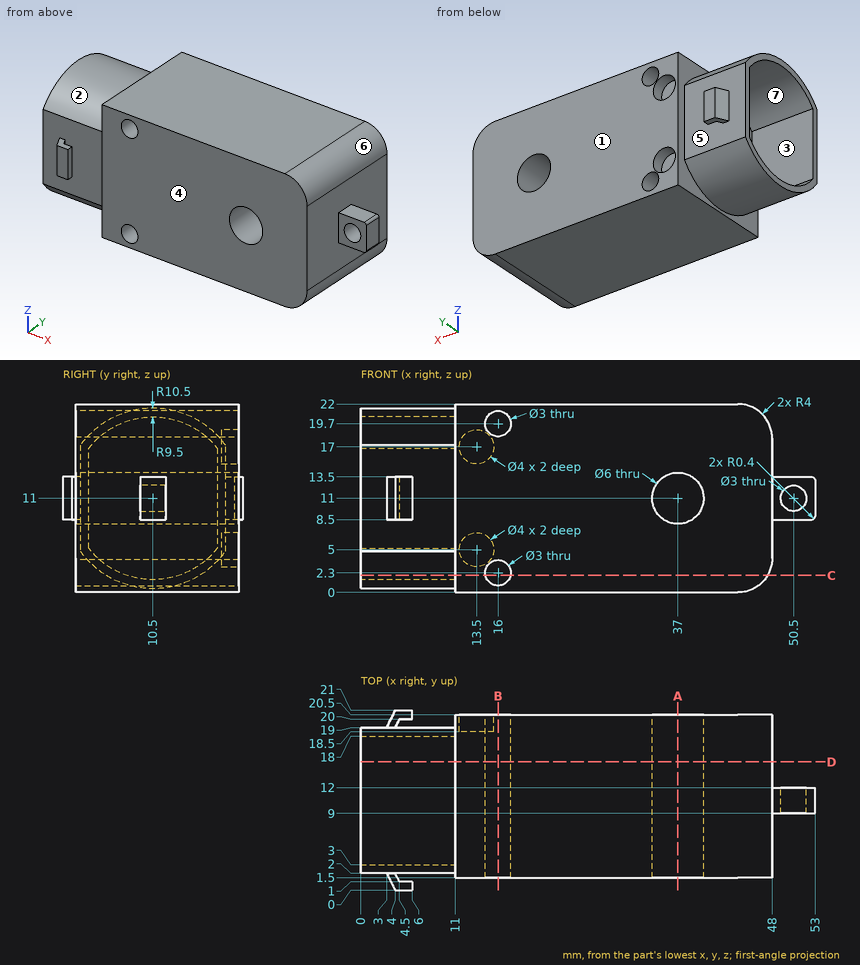
Print and shaded views of the part. All mm, measured from the part's lowest x, y and z. A direction names the side the tool comes from. Coordinates: 2 decimals unless noted, no trailing zeros. Loops run counter-clockwise (first coordinate to the right, second up) from the corner with the lowest first, then second, coordinate; pieces in that order, holes last. Notation, with made-up numbers: (80.5, 38) -> (138.5, 38) arc R27 ccw to (138.5, 76) -> close; hole circle Ø11 at (75, -35.5). An arc over 180 degrees is marked (long way). Use a Markdown table: item, result. Add a question column.
Item 1: Band-saw the part on B-B on x = 16. Write the cut outline in (y, z).
Item 2: Which spindle directions (+Z, -Z, +X, -X, +Y, -Y) get a long thin tool onto all of the face, cutting with end or side? Do the marked faces 1, 2, 3 and 4. Say none if no direction does.
Item 3: Band-saw the part on A-A on x = 37. Write the cut outline in (y, z).
Item 4: Probe probe 1 along X at (y, z) = (11.2, 11); probe 2 along X at (y, z) = (19.2, 17); probe 3 along X at (y, z) = (13.25, 5.25). List the from-to ranges inside material, lowest first.
Item 5: Band-saw the part on D-D on y = 15. Write the cut outline in (x, z).
Item 6: Flat gauge pins, fed straight in: P1, Ø2, axis at x = 13.5, z = 4.5, coming from the +Y side; P2, Ø2.5, axis at x = 51.5, z = 11.5, coming from the +Y side; P3, Ø0.9, axis at x = 51, y = 11, coming from the +Z side. Where does each tip first touch, or does it go through?
Item 7: Band-saw the part on C-C on z = 2. Write the cut outline in (x, y).
Item 8: Pull direction X, two halves, no side cores. Call the marked faces 5, 6 and 7: +X half, -X half, draft (parallel to the pull), parting line (faces both ways), or undercut.
Geometry says:
| question | item | result |
|---|---|---|
| 1 | outline | (1.5, 0) -> (20.5, 0) -> (20.5, 0.8) -> (1.5, 0.8) -> close; (1.5, 3.8) -> (20.5, 3.8) -> (20.5, 18.2) -> (1.5, 18.2) -> close; (1.5, 21.2) -> (20.5, 21.2) -> (20.5, 22) -> (1.5, 22) -> close |
| 2 | face 1 | +Z, -Z, +X, +Y |
| 2 | face 2 | +Z, -X |
| 2 | face 3 | -X |
| 2 | face 4 | +Z, -Z, +X, -Y |
| 3 | outline | (1.5, 0) -> (20.5, 0) -> (20.5, 8) -> (1.5, 8) -> close; (1.5, 14) -> (20.5, 14) -> (20.5, 22) -> (1.5, 22) -> close |
| 4 | probe 1 | 11 to 34, 40 to 49, 52 to 53 |
| 4 | probe 2 | 11 to 11.5, 15.5 to 48 |
| 4 | probe 3 | 11 to 48 |
| 5 | outline | (0, 1.51) -> (11, 1.51) -> (11, 0) -> (44, 0) arc R4 ccw to (48, 4) -> (48, 18) arc R4 ccw to (44, 22) -> (11, 22) -> (11, 20.49) -> (0, 20.49) -> (0, 19.37) -> (11, 19.37) -> (11, 2.63) -> (0, 2.63) -> close; hole circle Ø3 at (16, 2.3); hole circle Ø3 at (16, 19.7); hole circle Ø6 at (37, 11) |
| 6 | P1 | y = 18.5 |
| 6 | P2 | y = 12 |
| 6 | P3 | z = 13.5 |
| 7 | outline | (0, 5.09) -> (11, 5.09) -> (11, 1.5) -> (14.53, 1.5) -> (14.53, 20.5) -> (11, 20.5) -> (11, 15.91) -> (0, 15.91) -> (0, 13.54) -> (11, 13.54) -> (11, 7.46) -> (0, 7.46) -> close; (17.47, 1.5) -> (47.46, 1.5) -> (47.46, 20.5) -> (17.47, 20.5) -> close |
| 8 | face 5 | undercut |
| 8 | face 6 | +X half |
| 8 | face 7 | draft |
